Design review of the part shown in the three views and the two pictorial views. Dimensions are in mm from the part's minimum x, y and z. A direction names the side the tool comes from. Coordinates: 2 decimals unless noted, no trailing zeros. Write each loop counter-clockwise with the first axis right and the second up, starting at its lowest first coordinate (ties: lowest second). Pieces come first, ordered by that corner, then holes. Notation, with made-up numbers: (-20.75, 51.25) -> (-16.75, 51.25) arc R28 cw to (-16.75, 89.25) -> close; hole circle Ø9 at (36.25, -2.5). An arc over 180 degrees is marked (long way). Answer in a Markdown table with one row per item. Add a question column.
Item 1: Take a section at C-C, the plane z = 43. Write out the cut boundary in (x, y), and give its area (3 significant figures).
Item 2: To check wall thickness, follow line 1 (X direction, y = 10, z = 42.5); line 2 (Z direction, x = 6.25, y = 15); line 3 (X direction, y = 8.25, z = 26). State the ranges of each line that lie inside material, in increasing order.
Item 3: For the marked faces 1 and 2, list the 3-axis set-ups (+Z, -Z, +X, -X, +Y, -Y) from which the entire face can be reached by the end or side of a thin tool; tool diameter is ignored.
Item 4: Take a section at B-B, the plane z = 64. Write out the cut boundary in (x, y), and give its area (3 significant figures).
Item 5: Take a section at A-A, the plane x = 10.03. Write out the cut boundary in (y, z).
Item 6: Clearance check with flat-ended pins moving along their axes: P1, Ø12, axis at y = 13, z = 29.5, coming from the -X side; P2, Ø1.5, axis at x = 9.5, y = 5, coming from the +Z side; P3, Ø8, axis at y = 16.5, z = 50.5, coming from the -X side. State where each tip first meets the part, or that it passes through.
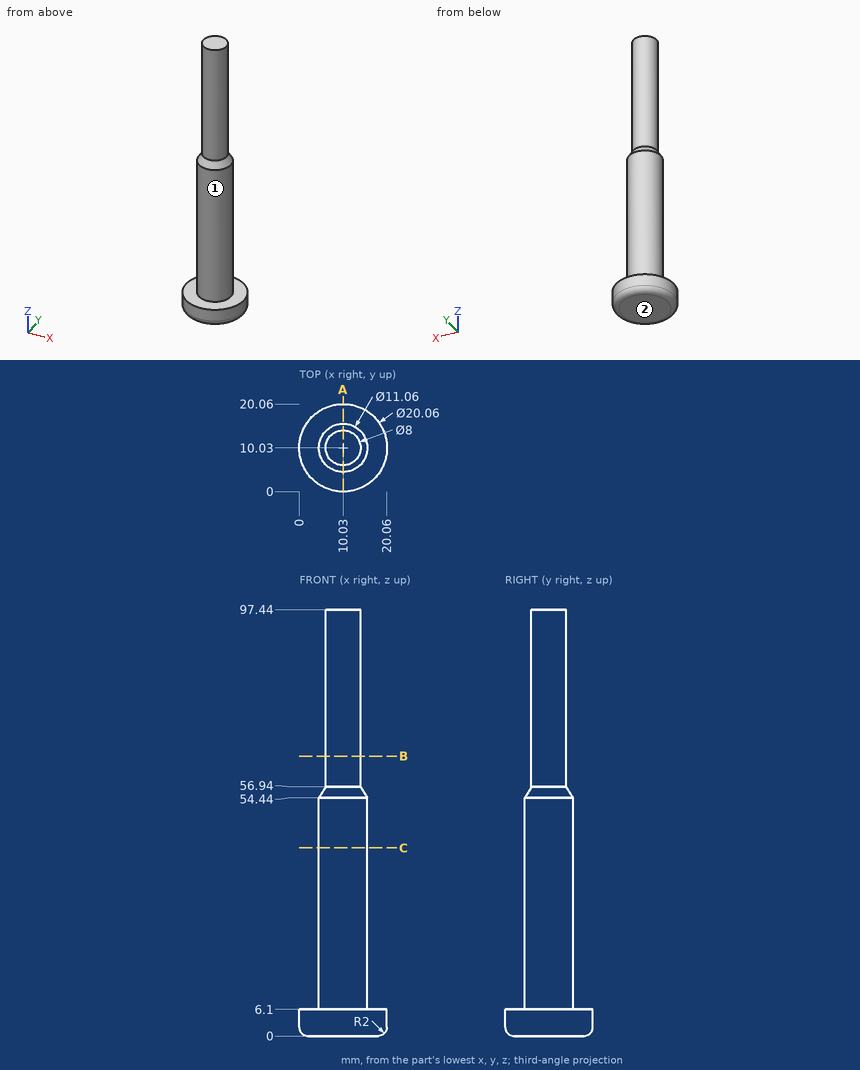
Answers:
| question | item | result |
|---|---|---|
| 1 | outline | circle Ø11.06 at (10.03, 10.03) |
| 1 | area | 96.1 mm^2 |
| 2 | line 1 | x = 4.5 to 15.56 |
| 2 | line 2 | z = 0 to 6.1 |
| 2 | line 3 | x = 4.79 to 15.27 |
| 3 | face 1 | +Z |
| 3 | face 2 | -Z, +X, -X, +Y, -Y |
| 4 | outline | circle Ø8 at (10.03, 10.03) |
| 4 | area | 50.3 mm^2 |
| 5 | outline | (0, 2) arc R2 ccw to (2, 0) -> (18.06, 0) arc R2 ccw to (20.06, 2) -> (20.06, 6.1) -> (15.56, 6.1) -> (15.56, 54.44) -> (14.03, 56.94) -> (14.03, 97.44) -> (6.03, 97.44) -> (6.03, 56.94) -> (4.5, 54.44) -> (4.5, 6.1) -> (0, 6.1) -> close |
| 6 | P1 | stops at x = 4.5 |
| 6 | P2 | stops at z = 56.44 |
| 6 | P3 | stops at x = 5.08 |
